```python
from build123d import *

# Parameters (mm, degrees)
SKETCH1_W            = 106
SKETCH1_H            = 106
MAINOUTLINE_DEPTH    = 1.6
RAILCUTOUTS_DEPTH    = 75.970394157
DOGBONES_DEPTH       = 75.970394157
SOLARFILLETS_DEPTH   = 75.970394157
HANDLINGFILLETS_R    = 1
M2_CLEARANCE_HOLE1_D = 2.1


with BuildPart() as part:
    # Sketch1 → mainOutline (new body)
    with BuildSketch(Plane.XY):
        Rectangle(SKETCH1_W, SKETCH1_H)
    extrude(amount=MAINOUTLINE_DEPTH)

    # Sketch4 → railCutouts (cut, through all)
    with BuildSketch(Plane(origin=(0, 0, 0), x_dir=(-1, 0, 0), z_dir=(0, 0, -1))):
        Polygon((-41.4, -41.4), (-48, -41.4), (-48, -39), (-49.9975, -39), (-60.106513243, -39), (-60.106513243, -61.452099286), (-39, -61.452099286), (-39, -49.9), (-39, -49), (-41.4, -49), align=None)
        Polygon((39, -56.27525328), (39, -49.9), (41.4, -49.9), (41.4, -41.4), (48, -41.4), (48, -40.5), (55.517672261, -40.5), (55.517672261, -56.27525328), align=None)
        Polygon((55.383846757, 40.5), (48, 40.5), (48, 41.4), (41.4, 41.4), (41.4, 49.9), (39, 49.9), (39, 57.687687567), (55.383846757, 57.687687567), align=None)
        Polygon((-39, 59.880423019), (-39, 49.9), (-39, 49), (-41.4, 49), (-41.4, 41.4), (-48, 41.4), (-48, 39), (-49.9975, 39), (-56.842822937, 39), (-56.842822937, 59.880423019), align=None)
    extrude(amount=-RAILCUTOUTS_DEPTH, mode=Mode.SUBTRACT)

    # Sketch5 → dogbones (cut, through all)
    with BuildSketch(Plane(origin=(0, 0, 0), x_dir=(-1, 0, 0), z_dir=(0, 0, -1))):
        with BuildLine():
            Line((-41.4, -43.196051224), (-44.546497129, -46.342548353))
            ThreePointArc((-44.546497129, -46.342548353), (-46.342548353, -46.342548353), (-46.342548353, -44.546497129))
            Line((-46.342548353, -44.546497129), (-43.196051224, -41.4))
            ThreePointArc((-43.196051224, -41.4), (-41.4, -41.4), (-41.4, -43.196051224))
        make_face()
        with BuildLine():
            Line((43.196051224, -41.4), (44.93821772, -43.142166495))
            ThreePointArc((44.93821772, -43.142166495), (44.93821772, -44.93821772), (43.142166495, -44.93821772))
            Line((43.142166495, -44.93821772), (41.4, -43.196051224))
            ThreePointArc((41.4, -43.196051224), (41.4, -41.4), (43.196051224, -41.4))
        make_face()
        with BuildLine():
            Line((41.4, 43.196051224), (43.13099025, 44.927041474))
            ThreePointArc((43.13099025, 44.927041474), (44.927041474, 44.927041474), (44.927041474, 43.13099025))
            Line((44.927041474, 43.13099025), (43.196051224, 41.4))
            ThreePointArc((43.196051224, 41.4), (41.4, 41.4), (41.4, 43.196051224))
        make_face()
        with BuildLine():
            Line((-43.196051224, 41.4), (-44.694846249, 42.898795025))
            ThreePointArc((-44.694846249, 42.898795025), (-44.694846249, 44.694846249), (-42.898795025, 44.694846249))
            Line((-42.898795025, 44.694846249), (-41.4, 43.196051224))
            ThreePointArc((-41.4, 43.196051224), (-41.4, 41.4), (-43.196051224, 41.4))
        make_face()
    extrude(amount=-DOGBONES_DEPTH, mode=Mode.SUBTRACT)

    # Sketch6 → solarFillets (cut, through all)
    with BuildSketch(Plane(origin=(0, 0, 0), x_dir=(-1, 0, 0), z_dir=(0, 0, -1))):
        with BuildLine():
            Line((-40, 50), (-40, 53))
            ThreePointArc((-40, 53), (-39, 54), (-38, 53))
            Line((-38, 53), (-38, 50))
            ThreePointArc((-38, 50), (-39, 49), (-40, 50))
        make_face()
        with BuildLine():
            Line((-49, 38), (-53, 38))
            ThreePointArc((-53, 38), (-54, 39), (-53, 40))
            Line((-53, 40), (-49, 40))
            ThreePointArc((-49, 40), (-48, 39), (-49, 38))
        make_face()
        with BuildLine():
            Line((-49, -40), (-55.214202913, -40))
            ThreePointArc((-55.214202913, -40), (-56.214202913, -39), (-55.214202913, -38))
            Line((-55.214202913, -38), (-49, -38))
            ThreePointArc((-49, -38), (-48, -39), (-49, -40))
        make_face()
        with BuildLine():
            Line((-38, -50), (-38, -53.916094318))
            ThreePointArc((-38, -53.916094318), (-39, -54.916094318), (-40, -53.916094318))
            Line((-40, -53.916094318), (-40, -50))
            ThreePointArc((-40, -50), (-39, -49), (-38, -50))
        make_face()
        with BuildLine():
            Line((40, -50.9), (40, -54.538013421))
            ThreePointArc((40, -54.538013421), (39, -55.538013421), (38, -54.538013421))
            Line((38, -54.538013421), (38, -50.9))
            ThreePointArc((38, -50.9), (39, -49.9), (40, -50.9))
        make_face()
        with BuildLine():
            Line((49, -39.5), (54.202622605, -39.5))
            ThreePointArc((54.202622605, -39.5), (55.202622605, -40.5), (54.202622605, -41.5))
            Line((54.202622605, -41.5), (49, -41.5))
            ThreePointArc((49, -41.5), (48, -40.5), (49, -39.5))
        make_face()
        with BuildLine():
            Line((49, 41.5), (54.556563772, 41.5))
            ThreePointArc((54.556563772, 41.5), (55.556563772, 40.5), (54.556563772, 39.5))
            Line((54.556563772, 39.5), (49, 39.5))
            ThreePointArc((49, 39.5), (48, 40.5), (49, 41.5))
        make_face()
        with BuildLine():
            Line((38, 50.9), (38, 55.828092709))
            ThreePointArc((38, 55.828092709), (39, 56.828092709), (40, 55.828092709))
            Line((40, 55.828092709), (40, 50.9))
            ThreePointArc((40, 50.9), (39, 49.9), (38, 50.9))
        make_face()
    extrude(amount=-SOLARFILLETS_DEPTH, mode=Mode.SUBTRACT)

    # handlingFillets
    handlingfillets_edges = [part.edges().sort_by_distance(p)[0] for p in [
        (-41.4, -49.9, 0.8),
        (-38, -53, 0.8),
        (-53, -39.5, 0.8),
        (-48, -41.4, 0.8),
        (-48, 41.4, 0.8),
        (-53, 39.5, 0.8),
        (-41.4, 49.9, 0.8),
        (-38, 53, 0.8),
        (38, 53, 0.8),
        (41.4, 49, 0.8),
        (48, 41.4, 0.8),
        (53, 38, 0.8),
        (53, -38, 0.8),
        (48, -41.4, 0.8),
        (41.4, -49, 0.8),
        (38, -53, 0.8),
    ]]
    fillet(handlingfillets_edges, radius=HANDLINGFILLETS_R)

    # M2 Clearance Hole1 (through all)
    with Locations(Plane(origin=(0, 0, 0), x_dir=(-1, 0, 0), z_dir=(0, 0, -1))):
        with Locations((50.5, -28), (28, -50.5), (-50.5, -28), (-28, -50.5), (-28, 50.5), (-50.5, 28), (28, 50.5), (50.5, 28)):
            Hole(M2_CLEARANCE_HOLE1_D / 2)


solid = part.part
```
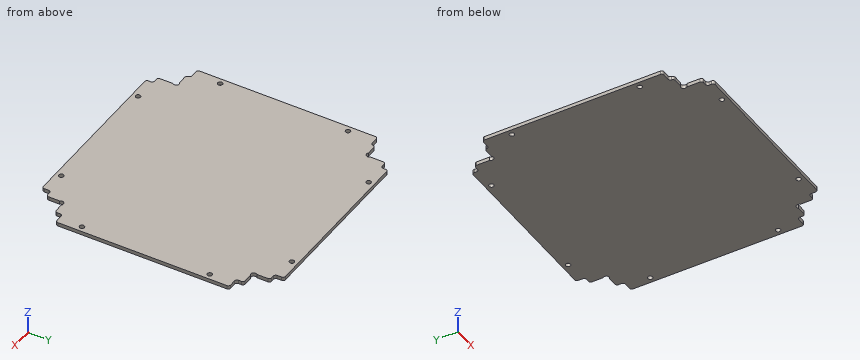
Part model, mm, in its own coordinate system. Round coordinates to 2 decimals unless told otherwise and drop trailing zeros.
Item 1: Probe L1, parallel to Y at x = -28, z = 0.85; L2, parallel to Y at x = 50.5, z = 1.1; L3, parallel to Y at x = 44, z = 1.45. List the from-to ranges inside material, lowest first.
Results:
L1: y = -53 to -51.55, -49.45 to 49.45, 51.55 to 53
L2: y = -38 to -29.05, -26.95 to 26.95, 29.05 to 38
L3: y = -41.4 to 41.4
Item 2: Cut at A-A, the plane z = 0.3. Count the separate pieces of the cut face and the enclosed holes in it, plus the area to 3 significant figures.
Results:
separate pieces: 1
enclosed holes: 8
area: 10,600 mm2
Item 3: Drop flat-ended pins along their axis: pin 1 Ø0.5 at (y, z) = (-51, 0.5) entering from +X; pin 2 Ø0.8 at (y, z) = (45.5, 1) entering from -X; pin 3 Ø0.8 at (y, z) = (-45.5, 0.5) entering from +X. Give the stop position or say it passes through.
Results:
pin 1: stops at x = 38
pin 2: stops at x = -41.4
pin 3: stops at x = 41.4
